Can you work these out from the drawing? Everything is in mm from the part's minimum corner. A direction names the side the tool comes from. Round coordinates to 2 decimals unless told otherwise and drop trailing zeros. Order: outer loops, then holes, each group sorted by start corner. A loop starts at its lowest first (then second) coordinate and runs counter-clockwise, first axis right, second up. Notation, with made-up numbers: (3, 78) - (23, 78) arc R37 ccw to (23, 116) - close; hole circle Ø4 at (75, -3.75). An arc over 180 degrees is marked (long way). Answer as a JSON object with one key per item and string values.
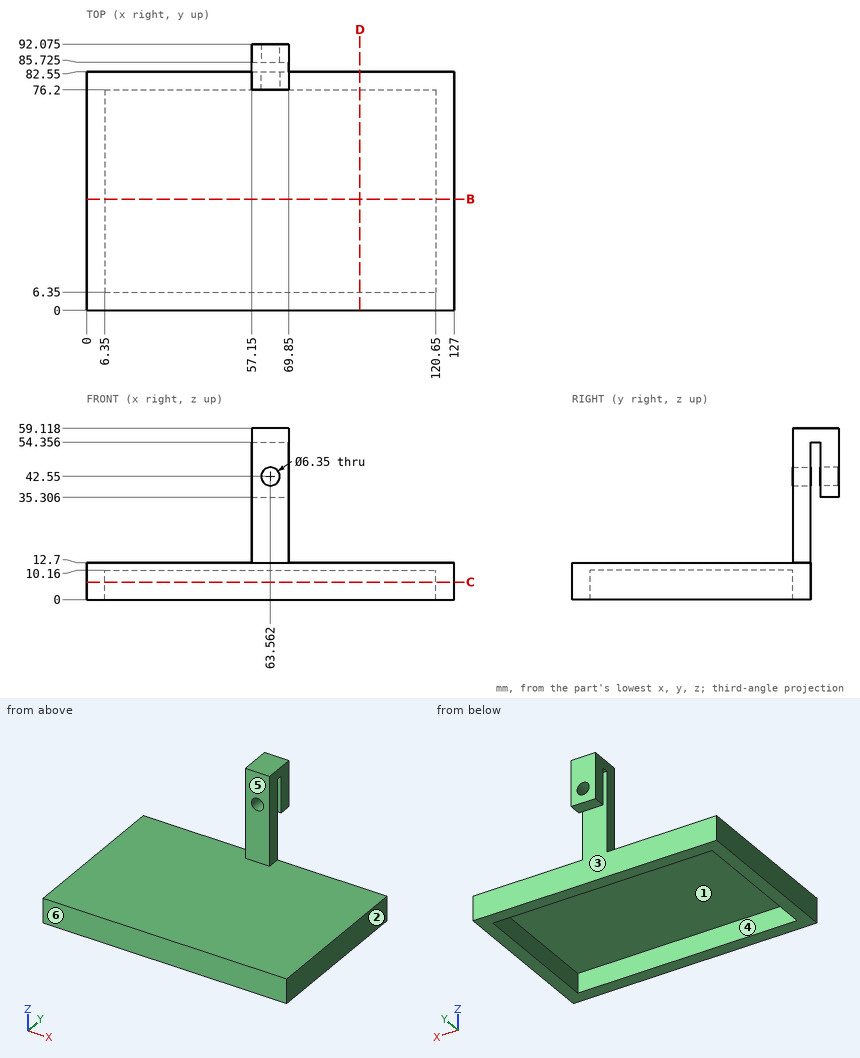
1. Imagine slicing it at C-C (z = 6). List the corners of the cut face in (x, y) for me.
Responses:
{"outline": "(0, 0) - (127, 0) - (127, 82.55) - (0, 82.55) - close; hole (6.35, 6.35) - (120.65, 6.35) - (120.65, 76.2) - (6.35, 76.2) - close"}
2. For the marked faces 4, 5 and 6, which set-ups out of +Z, -Z, +X, -X, +Y, -Y let a thin tool reach every point of the face, with its end or its side?
Responses:
{"face 4": "-Z", "face 5": "+Z, +X, -X, -Y", "face 6": "+Z, -Z, +X, -X, -Y"}
3. If I drill on L1, parallel to Y at x = 23, z = 5; L2, parallel to X at y = 12, z = 9; L3, parallel to Z at x = 53.5, y = 60.5, over which ranges is the centre line in solid material (lowest first)? Write a range as [from, to].
Responses:
{"L1": "[0, 6.35], [76.2, 82.55]", "L2": "[0, 6.35], [120.65, 127]", "L3": "[10.16, 12.7]"}
4. Thinking about a two-plate mould opening in X: for the marked faces 1, 2 and 3, which applies, pulls with the +X half, pulls with the -X half, needs draft (parallel to the pull), parting line crosses it, or undercut?
Responses:
{"face 1": "undercut", "face 2": "pulls with the +X half", "face 3": "needs draft"}
5. For P1, Ø6, axis at x = 35.5, y = 31, coming from the +Z side; P2, Ø3, axis at x = 75.5, z = 5.5, coming from the +Y side; P3, Ø10, axis at x = 65.5, z = 42, coming from the -Y side; P4, Ø5.5, axis at x = 63.56, z = 42.55, coming from the -Y side, each with a flat end and sliding along its axis, tell me the tip position at first contact or that it passes through.
Responses:
{"P1": "z = 12.7", "P2": "y = 82.55", "P3": "y = 76.2", "P4": "through"}
6. Imagine slicing it at B-B (y = 38.5). List the corners of the cut face in (x, z) for me.
Responses:
{"outline": "(0, 0) - (6.35, 0) - (6.35, 10.16) - (120.65, 10.16) - (120.65, 0) - (127, 0) - (127, 12.7) - (0, 12.7) - close"}
7. Imagine slicing it at D-D (x = 94.5). List the corners of the cut face in (y, z) for me.
Responses:
{"outline": "(0, 0) - (6.35, 0) - (6.35, 10.16) - (76.2, 10.16) - (76.2, 0) - (82.55, 0) - (82.55, 12.7) - (0, 12.7) - close"}
